Source: CAD feature listing. Evaluate the final solid. Frame: model axes, mm. Face numbers are marked on the shaded views. A direction names the side the tool comes from. Round coordinates to 2 decimals unless told otherwise and drop trailing zeros. Order: outer loops, then holes, each group sorted by start corner. A loop starts at its lowest first (then second) coordinate and runs counter-clockwise, first axis right, second up. Notation, with made-up numbers: (-25, -7.5) -> (6, -7.5) arc R10 cw to (6, 1.5) -> close; hole circle Ø10 at (17, 31). An arc over 180 degrees is marked (long way). One line per item, written item: value. Start each with the question number.
1) Reachability of the marked faces 1, 2 and 3 from +Z, -Z, +X, -X, +Y, -Y: full face, straight path, thin tool, end or side. Return the list, or none.
2) Ray query, L1, parallel to X at y = -4.5, z = 0; L2, parallel to X at y = -11, z = 0; L3, parallel to Y at x = -6.5, z = -5. Return the intervals inside material, ascending.
3) Mould query, pull axis Z, two halves, no side actions, for the marked faces 4, 5, 6 and 7. Classes: pulls with the +Z half, pulls with the -Z half, needs draft (parallel to the pull), parting line crosses it, or undercut.
4) Section B-B (y = -3.5). Return the cut outline in (x, z), and give its area (3 significant figures).
5) Pin query (flat end, axial travel): P1, Ø2, axis at x = -8, z = 4.5, coming from the -Y side; P2, Ø0.8, axis at y = 9, z = -16.5, coming from the -X side; P3, Ø2, axis at x = 1, y = 3.5, coming from the +Z side; P4, Ø4, axis at y = -13, z = 1.5, coming from the +X side. Return the tip coordinate at first contact, or that it passes through.
6) Section A-A (z = 1). Return the cut outline in (x, y).
7) Section D-D (y = 10.5). Return the cut outline in (x, z), and give its area (3 significant figures).
8) Section C-C (z = -11.5). Return the cut outline in (x, y).
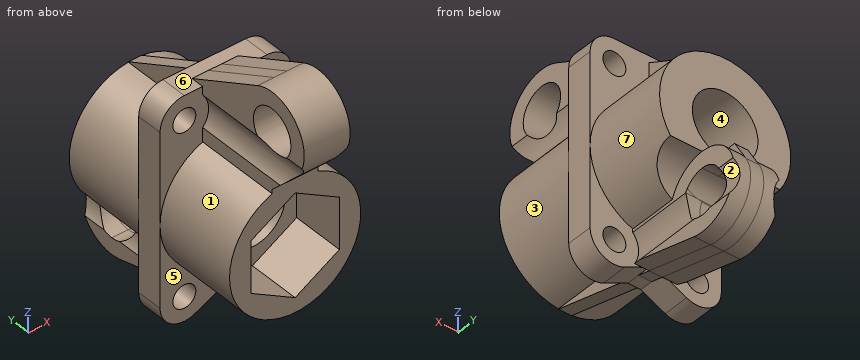
```python
from build123d import *
from build123d.topology import SkipClean

# Parameters (mm, degrees)
SKETCH2_R                = 10
BOSS_EXTRUDE1_DEPTH      = 15
SKETCH3_R                = 3.5
BOSS_EXTRUDE2_DEPTH      = 1
SKETCH6_R                = 1.75
BOSS_EXTRUDE3_DEPTH      = 2
SKETCH9_R                = 3.5
BOSS_EXTRUDE4_DEPTH      = 3.5
CUT_EXTRUDE12_DEPTH      = 7.2
CUT_EXTRUDE3_DEPTH       = 45.679413626
CUT_EXTRUDE3_DEPTH_BACK  = 8
SKETCH14_R               = 6
CUT_EXTRUDE7_DEPTH       = 35.978564903
SKETCH15_R               = 6
CUT_EXTRUDE8_DEPTH       = 33.94692706
CUT_EXTRUDE2_DEPTH       = 45.679413626
CUT_EXTRUDE2_DEPTH_BACK  = 45.679413626
SKETCH8_R                = 5
SKETCH16_R               = 3.7
CUT_EXTRUDE9_DEPTH       = 36.060661745
SKETCH17_R               = 3.7
CUT_EXTRUDE10_DEPTH      = 36.060661811
CUT_EXTRUDE13_DEPTH      = 34.782392028
CUT_EXTRUDE13_DEPTH_BACK = 34.782392028
SKETCH21_R               = 3.5


with BuildPart() as part:
    # Sketch2 → Boss-Extrude1 (new, symmetric)
    with BuildSketch(Plane(origin=(0, 0, 0), x_dir=(1, 0, 0), z_dir=(0, 1, 0))):
        with Locations(Location((0, 0, 0), (0, 0, 270))):
            Circle(SKETCH2_R)
    extrude(amount=BOSS_EXTRUDE1_DEPTH, both=True)

    # Sketch3 → Boss-Extrude2 (add, symmetric)
    with BuildSketch(Plane(origin=(0, 0, 0), x_dir=(0, 0, -1), z_dir=(1, 0, 0))):
        with BuildLine():
            Line((10, -15), (-10, -15))
            Line((-10, -15), (-14.264705882, -19.249974557))
            ThreePointArc((-14.264705882, -19.249974557), (-22.027248631, -19.853711682), (-23.850142927, -12.284126171))
            Line((-23.850142927, -12.284126171), (-10, 15))
            Line((-10, 15), (0, 15))
            Line((0, 15), (8.369565217, 20.118630488))
            ThreePointArc((8.369565217, 20.118630488), (15.066233626, 19.825140177), (17.311895323, 13.509405234))
            Line((17.311895323, 13.509405234), (10, -15))
        make_face()
        with Locations((11.5, 15)):
            Circle(SKETCH3_R, mode=Mode.SUBTRACT)
        with Locations((-18.5, -15)):
            Circle(SKETCH3_R, mode=Mode.SUBTRACT)
    extrude(amount=BOSS_EXTRUDE2_DEPTH, both=True)

    # Sketch6 → Boss-Extrude3 (add, symmetric)
    with BuildSketch(Plane(origin=(0, 0, 0), x_dir=(1, 0, 0), z_dir=(0, 1, 0))):
        with BuildLine():
            Line((-4.705422643, 15.616789864), (-1, 13.847096386))
            Line((-1, 13.847096386), (1, 13.847096386))
            Line((1, 13.847096386), (4.705422643, 15.616789864))
            ThreePointArc((4.705422643, 15.616789864), (8.273583515, 15.407720534), (10, 12.278029158))
            Line((10, 12.278029158), (10, -13.9143961))
            ThreePointArc((10, -13.9143961), (8.91629509, -16.530691191), (6.3, -17.6143961))
            Line((6.3, -17.6143961), (-6.3, -17.6143961))
            ThreePointArc((-6.3, -17.6143961), (-8.91629509, -16.530691191), (-10, -13.9143961))
            Line((-10, -13.9143961), (-10, 12.278029158))
            ThreePointArc((-10, 12.278029158), (-8.273583515, 15.407720534), (-4.705422643, 15.616789864))
        make_face()
        with Locations(Location((-6.3, 12.278029158, 0), (0, 0, 270))):
            Circle(SKETCH6_R, mode=Mode.SUBTRACT)
        with Locations(Location((6.3, 12.278029158, 0), (0, 0, 270))):
            Circle(SKETCH6_R, mode=Mode.SUBTRACT)
        with Locations(Location((6.3, -13.9143961, 0), (0, 0, 270))):
            Circle(SKETCH6_R, mode=Mode.SUBTRACT)
        with Locations(Location((-6.3, -13.9143961, 0), (0, 0, 270))):
            Circle(SKETCH6_R, mode=Mode.SUBTRACT)
    extrude(amount=BOSS_EXTRUDE3_DEPTH, both=True)

    # Sketch9 → Boss-Extrude4 (add, symmetric)
    # profile 1 of 2: a face of its own
    with BuildSketch(Plane(origin=(0, 0, 0), x_dir=(0, 0, -1), z_dir=(1, 0, 0))):
        with BuildLine():
            Line((14.360042571, 2), (17.311895323, 13.509405234))
            ThreePointArc((17.311895323, 13.509405234), (12.251208381, 20.952788084), (5.5, 15))
            Line((5.5, 15), (5.5, 2))
            Line((5.5, 2), (14.360042571, 2))
        make_face()
        with Locations((11.5, 15)):
            Circle(SKETCH9_R, mode=Mode.SUBTRACT)
    # profile 2 of 2: a face of its own
    with BuildSketch(Plane(origin=(0, 0, 0), x_dir=(0, 0, -1), z_dir=(1, 0, 0))):
        with BuildLine():
            Line((-23.850142927, -12.284126171), (-17.6143961, 0))
            Line((-17.6143961, 0), (-7.949874371, 0))
            Line((-7.949874371, 0), (-7.949874371, -15))
            Line((-7.949874371, -15), (-10, -15))
            Line((-10, -15), (-14.264705882, -19.249974557))
            ThreePointArc((-14.264705882, -19.249974557), (-22.027248631, -19.853711682), (-23.850142927, -12.284126171))
        make_face()
        with Locations((-18.5, -15)):
            Circle(SKETCH9_R, mode=Mode.SUBTRACT)
    extrude(amount=BOSS_EXTRUDE4_DEPTH, both=True)

    # Sketch20 → Cut-Extrude12 (cut)
    with BuildSketch(Plane(origin=(0, 0, 0), x_dir=(1, 0, 0), z_dir=(0, 1, 0))):
        Polygon((0, -7.794228634), (6.75, -3.897114317), (6.75, 3.897114317), (0, 7.794228634), (-6.75, 3.897114317), (-6.75, -3.897114317), align=None)
    extrude(amount=CUT_EXTRUDE12_DEPTH, mode=Mode.SUBTRACT)

    # Sketch10 → Cut-Extrude3 (cut, two sides: drawn at the far end of the back side and taken through both)
    with BuildSketch(Plane.XZ.offset(15).offset(-CUT_EXTRUDE3_DEPTH_BACK)):
        Polygon((0, -7.794228634), (6.75, -3.897114317), (6.75, 3.897114317), (0, 7.794228634), (-6.75, 3.897114317), (-6.75, -3.897114317), align=None)
    extrude(amount=CUT_EXTRUDE3_DEPTH + CUT_EXTRUDE3_DEPTH_BACK, mode=Mode.SUBTRACT)

    # Sketch14 → Cut-Extrude7 (cut, through all)
    with BuildSketch(Plane(origin=(-3.5, 0, 0), x_dir=(0, 0, -1), z_dir=(1, 0, 0))):
        with Locations((11.5, 15)):
            Circle(SKETCH14_R)
        with Locations((-18.5, -15)):
            Circle(SKETCH14_R)
    extrude(amount=-CUT_EXTRUDE7_DEPTH, mode=Mode.SUBTRACT)

    # Sketch15 → Cut-Extrude8 (cut, through all)
    with BuildSketch(Plane(origin=(3.5, 0, 3), x_dir=(0, 0, 1), z_dir=(-1, 0, 0))):
        with Locations((15.5, -15)):
            Circle(SKETCH15_R)
        with Locations((-14.5, 15)):
            Circle(SKETCH15_R)
    extrude(amount=-CUT_EXTRUDE8_DEPTH, mode=Mode.SUBTRACT)

    # Sketch8 → Cut-Extrude2 (cut, two sides: drawn at the far end of the back side and taken through both)
    with BuildSketch(Plane(origin=(0, 15, 0), x_dir=(1, 0, 0), z_dir=(0, 1, 0)).offset(-CUT_EXTRUDE2_DEPTH_BACK)):
        with Locations(Location((0, 0, 0), (0, 0, 270))):
            Circle(SKETCH8_R)
    extrude(amount=CUT_EXTRUDE2_DEPTH + CUT_EXTRUDE2_DEPTH_BACK, mode=Mode.SUBTRACT)

    # Sketch16 → Cut-Extrude9 (cut, through all)
    with BuildSketch(Plane(origin=(0, 2, 0), x_dir=(1, 0, 0), z_dir=(0, 1, 0))):
        with Locations((6.3, 12.278029158)):
            Circle(SKETCH16_R)
        with Locations((-6.3, 12.278029158)):
            Circle(SKETCH16_R)
    extrude(amount=CUT_EXTRUDE9_DEPTH, mode=Mode.SUBTRACT)

    # Sketch17 → Cut-Extrude10 (cut, through all)
    with BuildSketch(Plane.XZ.offset(2)):
        with Locations((6.3, 13.9143961)):
            Circle(SKETCH17_R)
        with Locations((-6.3, 13.9143961)):
            Circle(SKETCH17_R)
        with Locations((6.3, -12.278029158)):
            Circle(SKETCH17_R)
        with Locations((-6.3, -12.278029158)):
            Circle(SKETCH17_R)
    extrude(amount=CUT_EXTRUDE10_DEPTH, mode=Mode.SUBTRACT)

    # Sketch21 → Cut-Extrude13 (cut, two sides: drawn at the far end of the back side and taken through both)
    with SkipClean():  # the faces are left unmerged after this step: merging them gives an invalid solid
        with BuildSketch(Plane(origin=(0, 0, 0), x_dir=(0, 0, -1), z_dir=(1, 0, 0)).offset(-CUT_EXTRUDE13_DEPTH_BACK)):
            with Locations(Location((11.5, 15, 0), (0, 0, 242.046383782))):
                Circle(SKETCH21_R)
        extrude(amount=CUT_EXTRUDE13_DEPTH + CUT_EXTRUDE13_DEPTH_BACK, mode=Mode.SUBTRACT)


solid = part.part
```
Findings:
1. face 1: -X, -Y
1. face 2: +X, +Y
1. face 3: +X, -Y
2. L1: -10 to -5, 5 to 10
2. L2: -10 to -6.75, 6.75 to 10
2. L3: -15 to 15
3. face 4: undercut
3. face 5: needs draft
3. face 6: pulls with the +Z half
3. face 7: parting line crosses it
4. outline: (-3.5, 9.37) arc R10 ccw to (-1, -9.95) -> (-1, -12.95) -> (1, -12.95) -> (1, -9.95) arc R10 ccw to (3.5, 9.37) -> (3.5, 11.5) arc R3.7 cw to (3.5, 16.33) -> (3.5, 19.39) -> (-3.5, 19.39) -> (-3.5, 16.33) arc R3.7 cw to (-3.5, 11.5) -> close; hole circle Ø10 at (0, 0)
4. area: 303 mm2
5. P1: y = -15
5. P2: x = -3.5
5. P3: z = 16.35
5. P4: x = 10
6. outline: (-10, -2) -> (-9.95, -2) -> (-9.95, -15) -> (-6.75, -15) -> (-6.75, -7) -> (-4.9, -7) -> (-4.9, 0) -> (-6.75, 0) -> (-6.75, 7.2) -> (-4.9, 7.2) -> (-4.9, 15) -> (-9.95, 15) -> (-9.95, 2) -> (-10, 2) -> close; (4.9, -7) -> (6.75, -7) -> (6.75, -15) -> (9.95, -15) -> (9.95, -2) -> (10, -2) -> (10, 2) -> (9.95, 2) -> (9.95, 15) -> (4.9, 15) -> (4.9, 7.2) -> (6.75, 7.2) -> (6.75, 0) -> (4.9, 0) -> close
7. outline: (-6.58, -7.53) -> (-3.5, -7.53) -> (-3.5, -9.86) arc R3.7 cw to (-3.5, -14.7) -> (-3.5, -16.54) -> (3.5, -16.54) -> (3.5, -14.7) arc R3.7 cw to (3.5, -9.86) -> (3.5, -7.53) -> (6.58, -7.53) arc R10 ccw to (1, 9.95) -> (1, 12.28) -> (-1, 12.28) -> (-1, 9.95) arc R10 ccw to start; hole circle Ø10 at (0, 0)
7. area: 275 mm2
8. outline: (-10, -2) -> (-7.87, -2) -> (-7.87, 2) -> (-10, 2) -> close; (-4.73, -2) -> (-1, -2) -> (-1, -9.15) -> (1, -9.15) -> (1, -2) -> (4.73, -2) -> (4.73, 2) -> (2.68, 2) -> (2.68, 11.5) -> (-2.68, 11.5) -> (-2.68, 2) -> (-4.73, 2) -> close; (-2.68, 18.5) -> (2.68, 18.5) -> (2.68, 21) -> (-2.68, 21) -> close; (7.87, -2) -> (10, -2) -> (10, 2) -> (7.87, 2) -> close
